Design review of the part built by this model. Coordinates are the model's own, in mm. Face numbers are marked on the shaded views. Give positions to 0.01 mm unless a question says otherwise; leave off trailing zeros. Order: outer loops, then holes, each group sorted by start corner. A loop starts at its lowest first (then second) coordinate and runs counter-clockwise, first axis right, second up. Notation, with made-up numbers: (2.25, 71.5) -> (14.25, 71.5) arc R13 cw to (14.25, 79.5) -> close; hole circle Ø6 at (51.5, 17). An arc over 180 degrees is marked (long way). One line per item, written item: value.
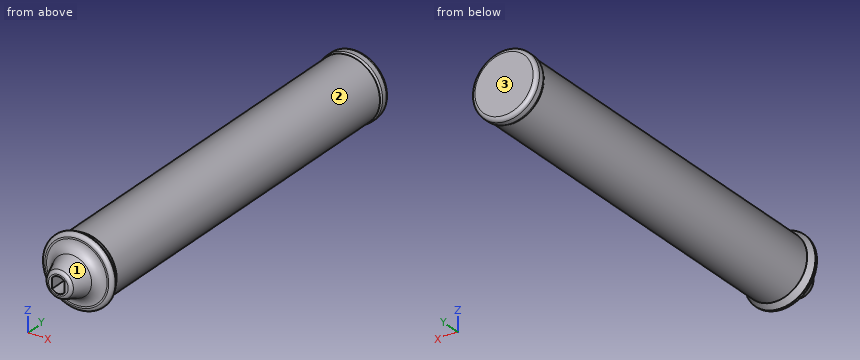
from build123d import *

# Parameters (mm, degrees)
SKETCH1_R           = 8.5
BOSS_EXTRUDE1_DEPTH = 100
SKETCH2_R           = 8.75
BOSS_EXTRUDE2_DEPTH = 3
FILLET5_R           = 1
FILLET8_R           = 1
SKETCH5_R           = 9.5
BOSS_EXTRUDE3_DEPTH = 3
FILLET10_R          = 1
CHAMFER2_SIZE2      = 1
CHAMFER2_SIZE       = 1.732050808
SKETCH6_R           = 6
BOSS_EXTRUDE4_DEPTH = 7
CUT_EXTRUDE1_DEPTH  = 7
CHAMFER4_SIZE2      = 2.687048245
CHAMFER4_SIZE       = 7
FILLET12_R          = 1


with BuildPart() as part:
    # Sketch1 → Boss-Extrude1 (new body)
    with BuildSketch(Plane(origin=(0, 0, 0), x_dir=(1, 0, 0), z_dir=(0, 1, 0))):
        with Locations(Location((0, 0, 0), (0, 0, 270))):
            Circle(SKETCH1_R)
    extrude(amount=BOSS_EXTRUDE1_DEPTH)

    # Sketch2 → Boss-Extrude2 (add)
    with BuildSketch(Plane(origin=(0, 100, 0), x_dir=(1, 0, 0), z_dir=(0, 1, 0))):
        with Locations(Location((0, 0, 0), (0, 0, 270))):
            Circle(SKETCH2_R)
    extrude(amount=BOSS_EXTRUDE2_DEPTH)

    # Fillet5
    fillet5_edges = [part.edges().sort_by_distance(p)[0] for p in [
        (0, 103, -8.75),
    ]]
    fillet(fillet5_edges, radius=FILLET5_R)

    # Fillet8
    # the kernel refuses this fillet: 1 mm, written as the material it takes off along each edge
    with BuildSketch(Plane(origin=(0, 100, 0), x_dir=(0, 0, 1), z_dir=(-1, 0, 0))) as fillet8_piece_1:
        with BuildLine():
            CenterArc((7.75, 0.661437828), FILLET8_R, 318.590377891, 41.409622109)
            Line((8.5, 0), (8.515, -0.013228757))
            ThreePointArc((8.515, -0.013228757), (8.625, -0.02), (8.75, -0.02))
            Line((8.75, -0.02), (8.77, 0))
            Line((8.77, 0), (8.77, 0.661437828))
            Line((8.77, 0.661437828), (8.75, 0.661437828))
        make_face()
    revolve(axis=Axis((0, 100, 0), (0, 1, 0)), mode=Mode.SUBTRACT)

    # Sketch5 → Boss-Extrude3 (add)
    with BuildSketch(Plane.XZ):
        with Locations(Location((0, 0, 0), (0, 0, 270))):
            Circle(SKETCH5_R)
    extrude(amount=BOSS_EXTRUDE3_DEPTH)

    # Fillet10
    fillet10_edges = [part.edges().sort_by_distance(p)[0] for p in [
        (0, -3, 9.5),
    ]]
    fillet(fillet10_edges, radius=FILLET10_R)

    # Chamfer2
    chamfer2_edges = [part.edges().sort_by_distance(p)[0] for p in [
        (0, 0, 9.5),
    ]]
    chamfer2_side = [part.faces().sort_by_distance(p)[0] for p in [
        (0, -0.02, 9.5),
    ]]
    chamfer(chamfer2_edges, length=CHAMFER2_SIZE - 0.0001, length2=CHAMFER2_SIZE2 - 0.0001, reference=chamfer2_side[0])  # a hair under: the kernel refuses the full size

    # Sketch6 → Boss-Extrude4 (add)
    with BuildSketch(Plane.XZ.offset(3)):
        with Locations(Location((0, 0, 0), (0, 0, 270))):
            Circle(SKETCH6_R)
    extrude(amount=BOSS_EXTRUDE4_DEPTH)

    # Sketch7 → Cut-Extrude1 (cut)
    with BuildSketch(Plane.XZ.offset(10)):
        with BuildLine():
            Line((-1.65, 1.378404875), (-1.65, -1.378404875))
            ThreePointArc((-1.65, -1.378404875), (0, -2.15), (1.65, -1.378404875))
            Line((1.65, -1.378404875), (1.65, 1.378404875))
            ThreePointArc((1.65, 1.378404875), (0, 2.15), (-1.65, 1.378404875))
        make_face()
    extrude(amount=-CUT_EXTRUDE1_DEPTH, mode=Mode.SUBTRACT)

    # Chamfer4
    chamfer4_edges = [part.edges().sort_by_distance(p)[0] for p in [
        (0, -10, 6),
    ]]
    chamfer4_side = [part.faces().sort_by_distance(p)[0] for p in [
        (0, -9.946259035, 6),
    ]]
    chamfer(chamfer4_edges, length=CHAMFER4_SIZE - 0.0001, length2=CHAMFER4_SIZE2 - 0.0001, reference=chamfer4_side[0])  # a hair under: the kernel refuses the full size

    # Fillet11: read off the stored shape, not the designer's step
    # Fillet11 outline → Fillet11 (revolve)
    with BuildSketch(Plane.XY):
        with BuildLine():
            Line((5.261101596, -3), (5.261101596, -4.924896151))
            ThreePointArc((5.261101596, -4.924896151), (6.362624165, -3.527621434), (8.061842876, -3))
            Line((8.061842876, -3), (5.261101596, -3))
        make_face()
    revolve(axis=Axis((0, 0, 0), (0, 1, 0)))

    # Fillet12
    fillet12_edges = [part.edges().sort_by_distance(p)[0] for p in [
        (0, -10, 3.313051755),
    ]]
    fillet(fillet12_edges, radius=FILLET12_R)


solid = part.part
Item 1: To check wall thickness, follow line 1 along Y through (x, z) = (-7.25, -4.5); line 2 along Z through (x, y) = (1, 71); line 3 along Y through (x, z) = (7.5, 2.75). State the ranges of each line that lie inside material, in increasing order. Write a range as from..to.
Returned:
line 1: -3..-0.06, 100.04..102.62
line 2: -8.44..8.44
line 3: -3..102.97
Item 2: Add section C-C on y = 83.5. Give the boundary of the cut face in (x, z).
Returned:
outline: circle Ø17 at (0, 0)
Item 3: Clearance check with flat-ended pins moving along their axes: P1, Ø6, axis at y = 74, z = -3.5, coming from the -X side; P2, Ø10, axis at x = -4.5, y = 46.5, coming from the +Z side; P3, Ø6, axis at y = 72, z = -4, coming from the +X side; P4, Ø2.5, axis at x = 0.5, z = 0.5, coming from the -Y side. State where each tip first meets the part, or that it passes through.
Returned:
P1: x = -8.49
P2: z = 8.5
P3: x = 8.44
P4: y = -10
Item 4: Draft analysis for pull direction Y (two halves, no side actions). For the marked faces 1, 2 and 3, state which applies: pulls with the +Y half, pulls with the -Y half, needs draft (parallel to the pull), parting line crosses it, or undercut.
Returned:
face 1: pulls with the -Y half
face 2: undercut
face 3: pulls with the +Y half
